Geometry check sheet. Reference: the model listing, model coordinates, mm. A direction names the side the tool comes from. Coordinates: 2 decimals unless noted, no trailing zeros. Order: outer loops, then holes, each group sorted by start corner. A loop starts at its lowest first (then second) coordinate and runs counter-clockwise, first axis right, second up. Notation, with made-up numbers: M 70.5,5.5 L 81.5,5.5 A12 ccw 81.5,18.5 Z; hole C -23.5,-38.75 d3. An arc over 180 degrees is marked long. One line per item, written item: value. Start each with the question number.
1) Draft check along Y on faces 1 (the cylindrical face through (3.35, -6.43, 2.46)), 2 (the flat face through (6, -6, 0)), 3 (the cylindrical face through (-1.73, -7.81, 11.01)). Enter one of: pulls with the +Y half, pulls with the -Y half, needs draft (parallel to the pull), parting line crosses it, or undercut.
2) Sectioned sample at A-A, the plane x = 0. Enter the section's corners in (y, z).
3) Sectioned sample at D-D, the plane y = 24. Enter the section's corners in (x, z).
4) Access from +Z, -Z, +X, -X, +Y, -Y to the whole of each face (thin tool, end or side, straight path). Record for faces 4 (the flat face through (0, -5, 5)), 5 (the flat face through (6, -6, 10)), 6 (the cylindrical face through (-4.296, 0.189, 8.451)).
5) Go/stop test with flat-tipped pins: P1, Ø5, axis at y = -18.5, z = 5, coming from the +X side; P2, Ø3, axis at y = 2.5, z = 9, coming from the -X side; P3, Ø3, axis at x = -9, y = -5.5, coming from the +Z side. Record where each tip stops, or that it passes through.
6) Sectioned sample at C-C, the plane z = 8.75. Enter the section's corners in (x, y).
7) Thickness scan on L1, parallel to Y at x = 0, z = 6.5; L2, parallel to Y at x = 0, z = 4.05; L3, parallel to Z at x = 1.5, y = -22.5. Record the ranges inside material, lowest first. Write a range as from..to.
```python
from build123d import *

# Parameters (mm, degrees)
SKETCH1_R           = 30
SKETCH1_R_2         = 4.3
BOSS_EXTRUDE1_DEPTH = 12
SKETCH2_R           = 7.25
CUT_EXTRUDE1_DEPTH  = 5
SKETCH3_R           = 30
SKETCH3_R_2         = 8
CUT_EXTRUDE2_DEPTH  = 2


with BuildPart() as part:
    # Sketch1 → Boss-Extrude1 (new body)
    with BuildSketch(Plane.XY):
        Circle(SKETCH1_R)
        Circle(SKETCH1_R_2, mode=Mode.SUBTRACT)
    extrude(amount=BOSS_EXTRUDE1_DEPTH)

    # Sketch2 → Cut-Extrude1 (cut)
    with BuildSketch(Plane.XY):
        Circle(SKETCH2_R)
    extrude(amount=CUT_EXTRUDE1_DEPTH, mode=Mode.SUBTRACT)

    # Sketch3 → Cut-Extrude2 (cut)
    with BuildSketch(Plane.XY.offset(12)):
        Circle(SKETCH3_R)
        Circle(SKETCH3_R_2, mode=Mode.SUBTRACT)
    extrude(amount=-CUT_EXTRUDE2_DEPTH, mode=Mode.SUBTRACT)


solid = part.part
```
Final values:
1. face 1: undercut
1. face 2: needs draft
1. face 3: parting line crosses it
2. outline: M -30,0 L -7.25,0 L -7.25,5 L -4.3,5 L -4.3,12 L -8,12 L -8,10 L -30,10 Z; M 4.3,5 L 7.25,5 L 7.25,0 L 30,0 L 30,10 L 8,10 L 8,12 L 4.3,12 Z
3. outline: M -18,0 L 18,0 L 18,10 L -18,10 Z
4. face 4: -Z
4. face 5: +Z
4. face 6: +Z, -Z
5. P1: stops at x = 25.38
5. P2: stops at x = -29.98
5. P3: stops at z = 10
6. outline: C 0,0 d60; hole C 0,0 d8.6
7. L1: y = -30..-4.3, 4.3..30
7. L2: y = -30..-7.25, 7.25..30
7. L3: z = 0..10
